Autodesk Inventor part; units mm, degrees
ref_plane "Work Plane1" through (-0.4516, -1.3897, 0) normal (-0.9511, 0.309, 0) x (0, 0, 1)
ref_plane "Work Plane2" through (0, 0, 29) normal (0, 0, 1) x (1, 0, 0)
ref_plane "YZ Plane" through (0, 0, 0) normal (1, 0, 0) x (0, 1, 0)
sketch "Sketch1" plane through (0, 0, 0) normal (0, 0, 1) x (1, 0, 0)
  circle A0 centre (0, 0) radius 17 construction
  circle A1 centre (0, 0) radius 8.5
  line L0 (-1.4613, 13.5) -> (1.43, 13.5)
  line L1 (1.43, 13.5) -> (1.43, 10.9067)
  line L2 (-1.4613, 10.9025) -> (-1.4613, 13.5)
  line L3 (-6.7782, 11.7623) -> (-5.2539, 9.6642)
  line L4 (-9.1173, 10.0628) -> (-6.7782, 11.7623)
  line L5 (-7.5905, 7.9614) -> (-9.1173, 10.0628)
  line L6 (-12.3974, 5.5317) -> (-9.931, 4.7303)
  line L7 (-13.2908, 2.782) -> (-12.3974, 5.5317)
  line L8 (-10.8205, 1.9793) -> (-13.2908, 2.782)
  line L9 (-13.2812, -2.8117) -> (-10.8147, -2.0103)
  line L10 (-12.3877, -5.5615) -> (-13.2812, -2.8117)
  line L11 (-9.9173, -4.7588) -> (-12.3877, -5.5615)
  line L12 (-9.092, -10.0812) -> (-7.5677, -7.9831)
  line L13 (-6.7529, -11.7806) -> (-9.092, -10.0812)
  line L14 (-5.2261, -9.6792) -> (-6.7529, -11.7806)
  line L15 (-1.43, -13.5) -> (-1.43, -10.9067)
  line L16 (1.4613, -13.5) -> (-1.43, -13.5)
  line L17 (1.4613, -10.9025) -> (1.4613, -13.5)
  line L18 (6.7782, -11.7623) -> (5.2539, -9.6642)
  line L19 (9.1173, -10.0628) -> (6.7782, -11.7623)
  line L20 (7.5905, -7.9614) -> (9.1173, -10.0628)
  line L21 (12.3974, -5.5317) -> (9.931, -4.7303)
  line L22 (13.2908, -2.782) -> (12.3974, -5.5317)
  line L23 (10.8205, -1.9793) -> (13.2908, -2.782)
  line L24 (13.2812, 2.8117) -> (10.8147, 2.0103)
  line L25 (12.3877, 5.5615) -> (13.2812, 2.8117)
  line L26 (9.9173, 4.7588) -> (12.3877, 5.5615)
  line L27 (9.092, 10.0812) -> (7.5677, 7.9831)
  line L28 (6.7529, 11.7806) -> (9.092, 10.0812)
  line L29 (5.2261, 9.6792) -> (6.7529, 11.7806)
  arc A2 (-1.4613, 10.9025) -> (-5.2539, 9.6642) centre (0, 0) ccw construction
  arc A3 (-1.4613, 10.9025) -> (-5.2539, 9.6642) centre (0, 0) ccw
  arc A4 (-7.5905, 7.9614) -> (-9.931, 4.7303) centre (0, 0) ccw
  arc A5 (-7.5905, 7.9614) -> (-9.931, 4.7303) centre (0, 0) ccw construction
  arc A6 (-10.8205, 1.9793) -> (-10.8147, -2.0103) centre (0, 0) ccw
  arc A7 (-10.8205, 1.9793) -> (-10.8147, -2.0103) centre (0, 0) ccw construction
  arc A8 (-9.9173, -4.7588) -> (-7.5677, -7.9831) centre (0, 0) ccw
  arc A9 (-9.9173, -4.7588) -> (-7.5677, -7.9831) centre (0, 0) ccw construction
  arc A10 (5.2261, 9.6792) -> (1.43, 10.9067) centre (0, 0) ccw construction
  arc A11 (5.2261, 9.6792) -> (1.43, 10.9067) centre (0, 0) ccw
  arc A12 (10.8205, -1.9793) -> (10.8147, 2.0103) centre (0, 0) ccw
  arc A13 (10.8205, -1.9793) -> (10.8147, 2.0103) centre (0, 0) ccw construction
  arc A14 (7.5905, -7.9614) -> (9.931, -4.7303) centre (0, 0) ccw
  arc A15 (7.5905, -7.9614) -> (9.931, -4.7303) centre (0, 0) ccw construction
  arc A16 (-5.2261, -9.6792) -> (-1.43, -10.9067) centre (0, 0) ccw
  arc A17 (1.4613, -10.9025) -> (5.2539, -9.6642) centre (0, 0) ccw
  arc A18 (-5.2261, -9.6792) -> (-1.43, -10.9067) centre (0, 0) ccw construction
  arc A19 (1.4613, -10.9025) -> (5.2539, -9.6642) centre (0, 0) ccw construction
  arc A20 (9.9173, 4.7588) -> (7.5677, 7.9831) centre (0, 0) ccw
  dimension "d5" = 360
  dimension "d14" = 5
  dimension "d15" = 11
  dimension "d16" = 34
  dimension "d17" = 17
  dimension "d24" = 2.5933
  dimension "d25" = 2.8912
extrude "Extrusion1" add sketch "Sketch1" along normal blind 29
sketch "Sketch2" plane through (0, 0, 29) normal (0, 0, 1) x (1, 0, 0)
  line L0 (-5.2539, 9.6642) -> (-6.7782, 11.7623)
  line L1 (-6.7782, 11.7623) -> (-9.1173, 10.0628)
  line L2 (-9.1173, 10.0628) -> (-7.5905, 7.9614)
  arc A0 (-7.5905, 7.9614) -> (-9.931, 4.7303) centre (0, 0) ccw
  line L3 (-9.931, 4.7303) -> (-12.3974, 5.5317)
  line L4 (-12.3974, 5.5317) -> (-13.2908, 2.782)
  line L5 (-13.2908, 2.782) -> (-10.8205, 1.9793)
  arc A1 (-10.8205, 1.9793) -> (-10.8147, -2.0103) centre (0, 0) ccw
  line L6 (-10.8147, -2.0103) -> (-13.2812, -2.8117)
  line L7 (-13.2812, -2.8117) -> (-12.3877, -5.5615)
  line L8 (-12.3877, -5.5615) -> (-9.9173, -4.7588)
  arc A2 (-9.9173, -4.7588) -> (-7.5677, -7.9831) centre (0, 0) ccw
  line L9 (-7.5677, -7.9831) -> (-9.092, -10.0812)
  line L10 (-9.092, -10.0812) -> (-6.7529, -11.7806)
  line L11 (-6.7529, -11.7806) -> (-5.2261, -9.6792)
  arc A3 (-5.2261, -9.6792) -> (-1.43, -10.9067) centre (0, 0) ccw
  line L12 (-1.43, -10.9067) -> (-1.43, -13.5)
  line L13 (-1.43, -13.5) -> (1.4613, -13.5)
  line L14 (1.4613, -13.5) -> (1.4613, -10.9025)
  arc A4 (1.4613, -10.9025) -> (5.2539, -9.6642) centre (0, 0) ccw
  line L15 (5.2539, -9.6642) -> (6.7782, -11.7623)
  line L16 (6.7782, -11.7623) -> (9.1173, -10.0628)
  line L17 (9.1173, -10.0628) -> (7.5905, -7.9614)
  arc A5 (7.5905, -7.9614) -> (9.931, -4.7303) centre (0, 0) ccw
  line L18 (9.931, -4.7303) -> (12.3974, -5.5317)
  line L19 (12.3974, -5.5317) -> (13.2908, -2.782)
  line L20 (13.2908, -2.782) -> (10.8205, -1.9793)
  arc A6 (10.8205, -1.9793) -> (10.8147, 2.0103) centre (0, 0) ccw
  line L21 (10.8147, 2.0103) -> (13.2812, 2.8117)
  line L22 (13.2812, 2.8117) -> (12.3877, 5.5615)
  line L23 (12.3877, 5.5615) -> (9.9173, 4.7588)
  arc A7 (9.9173, 4.7588) -> (7.5677, 7.9831) centre (0, 0) ccw
  line L24 (7.5677, 7.9831) -> (9.092, 10.0812)
  line L25 (9.092, 10.0812) -> (6.7529, 11.7806)
  line L26 (6.7529, 11.7806) -> (5.2261, 9.6792)
  arc A8 (5.2261, 9.6792) -> (1.43, 10.9067) centre (0, 0) ccw
  line L27 (1.43, 10.9067) -> (1.43, 13.5)
  line L28 (1.43, 13.5) -> (-1.4613, 13.5)
  line L29 (-1.4613, 13.5) -> (-1.4613, 10.9025)
  arc A9 (-1.4613, 10.9025) -> (-5.2539, 9.6642) centre (0, 0) ccw
  circle A10 centre (0, 0) radius 8.5
  circle A11 centre (0, 0) radius 8.5
extrude "Extrusion2" add sketch "Sketch2" against normal blind 11 contours A10
sketch "Sketch3" plane through (0, 0, 18) normal (0, 0, -1) x (-1, 0, 0)
  arc A0 (1.3217, 0.7094) -> (0.5581, -1.3923) centre (0, 0) ccw
  line L0 (0.5581, -1.3923) -> (1.3217, 0.7094)
  circle A1 centre (0, 0) radius 2.5
  point P0 (0, 0)
  dimension "d11" = 5
extrude "Extrusion3" add sketch "Sketch3" along normal blind 9
ref_plane "Work Plane1" through (-0.4516, -1.3897, 0) normal (-0.9511, 0.309, 0) x (0, 0, 1)
sketch "Sketch4" plane through (-0.4516, -1.3897, 0) normal (-0.9511, 0.309, 0) x (0, 0, 1)
  line L0 (31.9338, 1.727) -> (-3.3978, 1.727) construction
  point P0 (0, 1.4613)
ref_plane "Work Plane2" through (0, 0, 29) normal (0, 0, 1) x (1, 0, 0)
properties part number "felga"
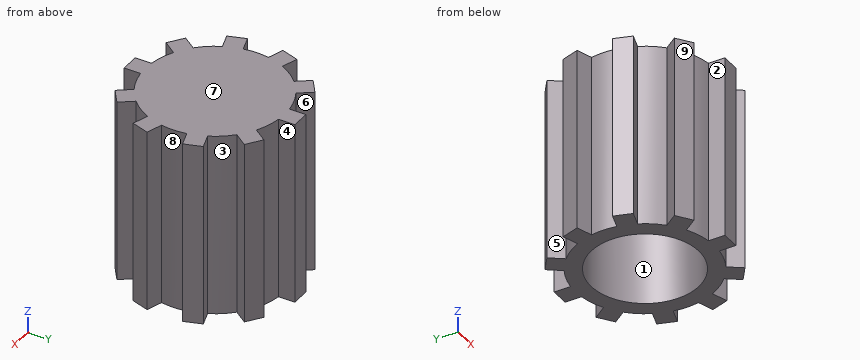
Build history of the part. All positions in model axes, mm. Face numbers are marked on the shaded views. A direction names the side the tool comes from. Coordinates: 2 decimals unless noted, no trailing zeros. Order: outer loops, then holes, each group sorted by start corner. A loop starts at its lowest first (then second) coordinate and runs counter-clockwise, first axis right, second up. Notation, with made-up numbers: M -22.75,-28.5 L 6.25,-28.5 A23 ccw 6.25,3.5 Z; hole C 9,-25 d3. An arc over 180 degrees is marked long. One line per question, with ' | ' between items. Start each with the question number.
1. Wall check: line 1 along Y through (x, z) = (0, 13.25); line 2 along X through (y, z) = (11, 6.25); line 3 along Z through (x, y) = (4.75, -7). Give the ranges that are in metal, low to high. Write a range as [from, to].
2. Cut at D-D (y = 7). Write the cut outline in (x, z).
3. Cut at A-A (z = 16). Count the separate pieces of the cut face and the enclosed holes in it, plus the area to 3 significant figures.
4. Flat gauge pins, fed straight in: P1, Ø1.3, axis at y = 11.5, z = 17.5, coming from the -X side; P2, Ø5, axis at x = 8, y = 9.5, coming from the -Z side; P3, Ø3, axis at y = -12, z = 15, coming from the -X side; P4, Ø3, axis at x = 0.5, y = 0, coming from the -Z side. Where does each tip first touch, or does it go through?
5. Mould opens along Y. For the marked faces 6, 7, 8 and 9 say: +Y half, -Y half, draft (parallel to the pull), parting line (faces both ways), or undercut.
6. Cut at B-B (x = 0). Write the cut outline in (y, z), plus the area to 3 significant figures.
7. Cut at C-C (y = 10.5). Write the cut outline in (x, z).
8. Tool access for the marked faces 1, 2, 3, 4 and 5: list every direction of +Z, -Z, +X, -X, +Y, -Y with a clear straight run to the whole face (end or side of a thin tool).
The answers:
1) line 1: y = [-13.5, -8.5], [-2.5, -1.5], [1.5, 2.5], [8.5, 13.5] | line 2: x = [-7.83, -6.22], [-1.46, 1.43], [6.19, 7.83] | line 3: z = [18, 29]
2) outline: M -8.49,0 L -4.82,0 L -4.82,18 L 4.82,18 L 4.82,0 L 8.49,0 L 8.49,29 L -8.49,29 Z
3) separate pieces: 2 | enclosed holes: 2 | area: 240 mm2
4) P1: stops at x = -8.03 | P2: stops at z = 0 | P3: stops at x = -8.52 | P4: stops at z = 9
5) face 6: +Y half | face 7: draft | face 8: undercut | face 9: -Y half
6) outline: M -13.5,0 L -8.5,0 L -8.5,18 L -2.5,18 L -2.5,9 L -1.5,9 L -1.5,18 L 1.5,18 L 1.5,9 L 2.5,9 L 2.5,18 L 8.5,18 L 8.5,0 L 13.5,0 L 13.5,29 L -13.5,29 Z | area: 495 mm2
7) outline: M -8.52,0 L -5.86,0 L -5.86,29 L -8.52,29 Z; M -3.28,0 L 3.28,0 L 3.28,29 L -3.28,29 Z; M 5.82,0 L 8.52,0 L 8.52,29 L 5.82,29 Z
8) face 1: -Z | face 2: +Z, -Z, -Y | face 3: +Z, -Z | face 4: +Z, -Z, +Y | face 5: +Z, -Z, -X
